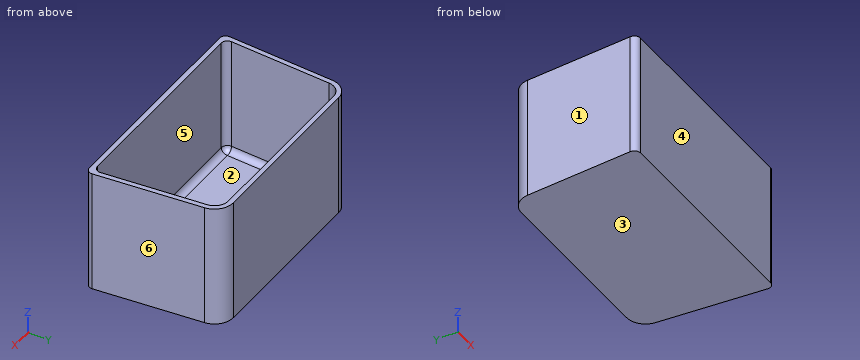
from build123d import *

# Parameters (mm, degrees)
F1_DEPTH = 100
F2_T     = -4
F3_R     = 5


with BuildPart() as f1:
    # F0 (on Top) → F1 (new body)
    with BuildSketch(Plane.XY):
        with BuildLine():
            Line((-74.9023482991, 51.9376612258), (-81.8753698939, -40.8005561921))
            Line((-81.8753698939, -40.8005561921), (105.1246301061, -40.8005561921))
            Line((105.1246301061, -40.8005561921), (98.1516085112, 51.9376612258))
            ThreePointArc((98.1516085112, 51.9376612258), (93.2625692956, 62.0850012182), (82.7772187745, 66.1994438079))
            Line((82.7772187745, 66.1994438079), (-59.5279585624, 66.1994438079))
            ThreePointArc((-59.5279585624, 66.1994438079), (-70.0133090834, 62.0850012182), (-74.9023482991, 51.9376612258))
        make_face()
    extrude(amount=F1_DEPTH)

    # F2
    f2_openings = [f1.faces().sort_by_distance(p)[0] for p in [
        (11.62463, 11.668388, 100),
    ]]
    offset(amount=F2_T, openings=f2_openings)

    # F3
    f3_edges = [f1.edges().sort_by_distance(p)[0] for p in [
        (105.12463, -40.800556, 50),
        (-81.87537, -40.800556, 50),
        (100.812577, -36.800556, 52),
        (-77.563317, -36.800556, 52),
        (11.62463, -36.800556, 4),
        (97.487723, 7.418595, 4),
    ]]
    fillet(f3_edges, radius=F3_R)


solid = f1.part
Check sheet for the modelled part. Datum: model origin and axes. Units: mm. Face numbers are marked on the shaded views. A direction names the side the tool comes from. Give positions to 0.01 mm unless a question says otherwise; leave off trailing zeros. Write each loop counter-clockwise with the first axis right and the second up, starting at its lowest first coordinate (ties: lowest second). Pieces come first, ordered by that corner, then holes. Notation, with made-up numbers: (10.5, 32.25) -> (25.5, 32.25) arc R15 cw to (25.5, 51.25) -> close; hole circle Ø11 at (77.5, -5). An arc over 180 degrees is marked (long way). One line per item, written item: value. Start each with the question number.
Item 1: Draft check along Y on the marked faces 1, 2, 3 and 4. Enter one of: +Y half, -Y half, draft (parallel to the pull), parting line (faces both ways), or undercut.
Item 2: Material ranges on probe 1 along Y at (x, z) = (-41, 31); probe 2 along X at (y, z) = (29, 70) (3 decimals); probe 3 along Z at (x, y) = (-5.5, 19.5), recorded low to high. Write a range as from..to.
Item 3: Tool access check on the marked faces 5 and 6. Record the directions out of +Z, -Z, +X, -X, +Y, -Y that give a thin tool (end or side, any length) a straight path to the whole face; none if there is none.
Item 4: Section check B-B on x = 3.5. Record the cut outline in (y, z), then the cut area to 3 significant figures.
Item 5: Gauge pin test, flat ends, axial feed: pin 1 (5 mm diameter, centred on y = 21.5, z = 12, fed in from +X); pin 2 (6 mm diameter, centred on y = 10.5, z = 29.5, fed in from +X); pin 3 (6 mm diameter, centred on y = -12, z = 40.5, fed in from -X). Record the tip position at first contact, or that the pin passes through.
Item 6: Section check A-A on z = 63.5. Record the cut outline in (x, y).
Results list:
1. face 1: +Y half
1. face 2: undercut
1. face 3: draft
1. face 4: -Y half
2. probe 1: -40.8..-36.8, 62.2..66.2
2. probe 2: -76.627..-72.616, 95.865..99.876
2. probe 3: 0..4
3. face 5: +Z
3. face 6: +Z, -Z, +X, +Y
4. outline: (-40.8, 0) -> (66.2, 0) -> (66.2, 100) -> (62.2, 100) -> (62.2, 9) arc R5 cw to (57.2, 4) -> (-31.8, 4) arc R5 cw to (-36.8, 9) -> (-36.8, 100) -> (-40.8, 100) -> close
4. area: 1,210 mm²
5. pin 1: x = 100.63
5. pin 2: x = 101.49
5. pin 3: x = -79.94
6. outline: (-81.47, -35.43) arc R5 ccw to (-76.49, -40.8) -> (99.73, -40.8) arc R5 ccw to (104.72, -35.43) -> (98.15, 51.94) arc R15.42 ccw to (82.78, 66.2) -> (-59.53, 66.2) arc R15.42 ccw to (-74.9, 51.94) -> close; hole (-77.16, -31.43) arc R5 ccw to (-72.17, -36.8) -> (95.42, -36.8) arc R5 ccw to (100.41, -31.43) -> (94.16, 51.64) arc R11.42 ccw to (82.78, 62.2) -> (-59.53, 62.2) arc R11.42 ccw to (-70.91, 51.64) -> close
